Geometry: final body of the model. Coordinates: model frame, mm. A direction names the side the tool comes from. Coordinates: 2 decimals unless noted, no trailing zeros. Loops run counter-clockwise (first coordinate to the right, second up) from the corner with the lowest first, then second, coordinate; pieces in that order, holes last. Notation, with made-up numbers: (42, 15) - (59, 15) arc R31 cw to (59, 45) - close; hole circle Ø5 at (40, -4). An arc over 180 degrees is marked (long way). Return JSON: item names as keys, results as strings.
from build123d import *

# Parameters (mm, degrees)
BOSS_EXTRUDE1_DEPTH     = 9.525
SKETCH2_W               = 94.331668948
SKETCH2_H               = 25.4
CUT_EXTRUDE1_DEPTH      = 10.525
FILLET1_R               = 6.35
FILLET2_R               = 6.35
F_1_4_CLEARANCE_HOLE1_D = 6.7564
SKETCH5_W               = 19.685
SKETCH5_H               = 12.7
CUT_EXTRUDE2_DEPTH      = 10.525
FILLET3_R               = 6.35
CUT_EXTRUDE3_DEPTH      = 10.525
FILLET4_R               = 12.7
FILLET5_R               = 6.35


with BuildPart() as part:
    # Sketch1 → Boss-Extrude1 (new body)
    with BuildSketch(Plane(origin=(0, 0, 0), x_dir=(1, 0, 0), z_dir=(0, 1, 0))):
        with BuildLine():
            Line((28.575, 81.75625), (28.575, 160.782))
            Line((28.575, 160.782), (0, 160.782))
            Line((0, 160.782), (0, 0))
            Line((0, 0), (82.55, 0))
            Line((82.55, 0), (118.11, 120.65))
            Line((118.11, 120.65), (118.11, 139.7))
            ThreePointArc((118.11, 139.7), (139.7, 161.29), (161.29, 139.7))
            Line((161.29, 139.7), (161.29, 120.65))
            Line((161.29, 120.65), (180.975, 120.65))
            Line((180.975, 120.65), (180.975, 139.7))
            Line((180.975, 139.7), (180.975, 177.8))
            Line((180.975, 177.8), (121.7041, 177.8))
            Line((121.7041, 177.8), (80.9625, 177.8))
            Line((80.9625, 177.8), (80.9625, 81.75625))
            ThreePointArc((80.9625, 81.75625), (54.76875, 55.5625), (28.575, 81.75625))
        make_face()
    extrude(amount=BOSS_EXTRUDE1_DEPTH)

    # Sketch2 → Cut-Extrude1 (cut, through all)
    with BuildSketch(Plane(origin=(0, 9.525, 0), x_dir=(1, 0, 0), z_dir=(0, 1, 0))):
        with Locations((47.165834474, 12.7)):
            Rectangle(SKETCH2_W, SKETCH2_H)
    extrude(amount=-CUT_EXTRUDE1_DEPTH, mode=Mode.SUBTRACT)

    # Fillet1
    fillet1_edges = [part.edges().sort_by_distance(p)[0] for p in [
        (0, 4.7625, -25.4),
    ]]
    fillet(fillet1_edges, radius=FILLET1_R)

    # Fillet2
    fillet2_edges = [part.edges().sort_by_distance(p)[0] for p in [
        (0, 4.7625, -160.782),
        (180.975, 4.7625, -177.8),
        (180.975, 4.7625, -120.65),
        (90.036315789, 4.7625, -25.4),
    ]]
    fillet(fillet2_edges, radius=FILLET2_R)

    # 1/4 Clearance Hole1 (through all)
    with Locations(Plane(origin=(0, 9.525, 0), x_dir=(1, 0, 0), z_dir=(0, 1, 0))):
        with Locations((14.2875, 146.05), (14.2875, 44.45), (99.2378, 146.05), (170.92295, 146.05)):
            Hole(F_1_4_CLEARANCE_HOLE1_D / 2)

    # Sketch5 → Cut-Extrude2 (cut, through all)
    with BuildSketch(Plane(origin=(0, 9.525, 0), x_dir=(1, 0, 0), z_dir=(0, 1, 0))):
        with Locations((171.1325, 127)):
            Rectangle(SKETCH5_W, SKETCH5_H)
    extrude(amount=-CUT_EXTRUDE2_DEPTH, mode=Mode.SUBTRACT)

    # Fillet3
    fillet3_edges = [part.edges().sort_by_distance(p)[0] for p in [
        (180.975, 4.7625, -133.35),
    ]]
    fillet(fillet3_edges, radius=FILLET3_R)

    # Sketch6 → Cut-Extrude3 (cut, through all)
    with BuildSketch(Plane(origin=(0, 9.525, 0), x_dir=(1, 0, 0), z_dir=(0, 1, 0))):
        with BuildLine():
            Line((26.486121599, 81.75625), (26.486121599, 177.8))
            Line((26.486121599, 177.8), (83.051378401, 177.8))
            Line((83.051378401, 177.8), (83.051378401, 81.75625))
            ThreePointArc((83.051378401, 81.75625), (54.76875, 53.473621599), (26.486121599, 81.75625))
        make_face()
    extrude(amount=-CUT_EXTRUDE3_DEPTH, mode=Mode.SUBTRACT)

    # Fillet4
    fillet4_edges = [part.edges().sort_by_distance(p)[0] for p in [
        (161.29, 4.7625, -133.35),
    ]]
    fillet(fillet4_edges, radius=FILLET4_R)

    # Fillet5
    fillet5_edges = [part.edges().sort_by_distance(p)[0] for p in [
        (26.486121599, 4.7625, -160.782),
        (83.051378401, 4.7625, -177.8),
    ]]
    fillet(fillet5_edges, radius=FILLET5_R)


solid = part.part
Item 1: Section query B-B, the plane y = 5.75. Count the separate pieces of the cut face and the enclosed holes in it, and give its area (3 significant figures).
Worked out:
{"separate pieces": "1", "enclosed holes": "4", "area": "11,100 mm^2"}
Item 2: Mould query, pull axis X, two halves, no side actions, for faces 1 (the face through (89, 0, -103)), 2 (the face through (84.96, 4.7, -175.99)), 3 (the face through (15.02, 4.696, -142.752)). Classes: +X half, -X half, draft (parallel to the pull), parting line (faces both ways), or undercut.
Worked out:
{"face 1": "draft", "face 2": "-X half", "face 3": "undercut"}
Item 3: Reachability of faces 4 (the face through (13, 5, -160.782)), 5 (the face through (26.486, 5, -118)), 6 (the face through (173.6, 4.7, -143.99)) from +Z, -Z, +X, -X, +Y, -Y: full face, straight path, thin tool, end or side. Return the list, or none.
Worked out:
{"face 4": "-Z, -X, +Y, -Y", "face 5": "-Z, +Y, -Y", "face 6": "+Y, -Y"}
Item 4: Ray query, probe 1 along X at (y, z) = (7.5, -146.05) (3 decimals); probe 2 along X at (y, z) = (3.5, -127); probe 3 along X at (y, z) = (6.25, -60). Return the intervals inside material, ascending. Write a range as from..to.
Worked out:
{"probe 1": "0..10.909, 17.666..26.486, 83.051..95.86, 102.616..119.065, 160.335..167.545, 174.301..180.975", "probe 2": "0..26.49, 83.05..118.11", "probe 3": "0..36.7, 72.84..100.23"}
Item 5: Section query D-D, the plane z = -44.45. Return loops of the section in (x, y) (3 decimals), and give its area (3 significant figures).
Worked out:
{"outline": "(0, 0) - (10.909, 0) - (10.909, 9.525) - (0, 9.525) - close; (17.666, 0) - (95.651, 0) - (95.651, 9.525) - (17.666, 9.525) - close", "area": "847 mm^2"}
Item 6: Section query A-A, the plane z = -74. Return loops of the section in (x, y) (3 decimals), and give its area (3 significant figures).
Worked out:
{"outline": "(0, 0) - (27.57, 0) - (27.57, 9.525) - (0, 9.525) - close; (81.967, 0) - (104.361, 0) - (104.361, 9.525) - (81.967, 9.525) - close", "area": "476 mm^2"}
Item 7: First-contact query: pin 1 Ø5 at (y, z) = (8, -46.5) entering from +X; pin 2 Ø1.4 at (x, y) = (174, 5) entering from +Z; pin 3 Ø5.5 at (x, z) = (99.24, -146.05) entering from -Y; pin 4 Ø5 at (x, y) = (12.5, 7) entering from -Z. Flat tips, straight axial feed; report the tip coordinate or a pass-through.
Worked out:
{"pin 1": "x = 96.99", "pin 2": "z = -133.35", "pin 3": "through", "pin 4": "z = -160.78"}
Item 8: Section query C-C, the plane z = -146.05. Return loops of the section in (x, y) (3 decimals).
Worked out:
{"outline": "(0, 0) - (10.909, 0) - (10.909, 9.525) - (0, 9.525) - close; (17.666, 0) - (26.486, 0) - (26.486, 9.525) - (17.666, 9.525) - close; (83.051, 0) - (95.86, 0) - (95.86, 9.525) - (83.051, 9.525) - close; (102.616, 0) - (119.065, 0) - (119.065, 9.525) - (102.616, 9.525) - close; (160.335, 0) - (167.545, 0) - (167.545, 9.525) - (160.335, 9.525) - close; (174.301, 0) - (180.975, 0) - (180.975, 9.525) - (174.301, 9.525) - close"}
